```python
from build123d import *

# Parameters (mm, degrees)
F0_W      = 171
F0_H      = 141
F1_DEPTH  = 40
F2_W      = 82.5
F2_H      = 67.5
F3_DEPTH  = 3
F4_W      = 80.5
F4_H      = 65.5
F5_DEPTH  = 3
F6_W      = 82.5
F6_H      = 67.5
F7_DEPTH  = 36
F9_START  = 30
F9_DEPTH  = 6
F11_DEPTH = 39.9
F12_R     = 2.99999
F13_R     = 2.99999
F15_DEPTH = 87.6
F17_DEPTH = 58
F19_DEPTH = 2.5
F20_W     = 34
F20_H     = 30
F20_H_2   = 5
F21_DEPTH = 1.5
F22_W     = 22
F22_H     = 36
F23_DEPTH = 1
F25_DEPTH = 107.7
F27_DEPTH = 2
F29_DEPTH = 18
F31_DEPTH = 6
F33_DEPTH = 6


# Not quite as in the source:
# - a fillet or chamfer is up to 0.001 mm smaller than in the source, because OpenCascade refuses the exact size


with BuildPart() as f1:
    # F0 (on Front) → F1 (new body)
    with BuildSketch(Plane.XZ):
        with Locations((85.5, 70.5)):
            Rectangle(F0_W, F0_H)
    extrude(amount=F1_DEPTH)

    # F2 (on face) → F3 (cut)
    with BuildSketch(Plane.XZ.offset(40)):
        with Locations((126.75, 104.25)):
            Rectangle(F2_W, F2_H)
        with Locations((44.25, 104.25)):
            Rectangle(F2_W, F2_H)
        with Locations((126.75, 36.75)):
            Rectangle(F2_W, F2_H)
        with Locations((44.25, 36.75)):
            Rectangle(F2_W, F2_H)
    extrude(amount=-F3_DEPTH, mode=Mode.SUBTRACT)

    # F4 (on face) → F5 (cut)
    with BuildSketch(Plane.XZ.offset(37)):
        with Locations((45.25, 103.25)):
            Rectangle(F4_W, F4_H)
        with Locations((125.75, 103.25)):
            Rectangle(F4_W, F4_H)
        with Locations((125.75, 37.75)):
            Rectangle(F4_W, F4_H)
        with Locations((45.25, 37.75)):
            Rectangle(F4_W, F4_H)
    extrude(amount=-F5_DEPTH, mode=Mode.SUBTRACT)

    # F6 (on face) → F7 (cut)
    with BuildSketch(Plane.XZ.offset(37)):
        with Locations((126.75, 104.25)):
            Rectangle(F6_W, F6_H)
        with Locations((44.25, 104.25)):
            Rectangle(F6_W, F6_H)
        with Locations((126.75, 36.75)):
            Rectangle(F6_W, F6_H)
        with Locations((44.25, 36.75)):
            Rectangle(F6_W, F6_H)
    extrude(amount=-F7_DEPTH, mode=Mode.SUBTRACT)

    # F8 (on face) → F9 (join)
    with BuildSketch(Plane.XZ.offset(1).offset(F9_START)):
        Polygon((3, 138), (3, 70.5), (6, 70.5), (6, 135), (85.5, 135), (85.5, 138), align=None)
        Polygon((3, 70.5), (3, 3), (85.5, 3), (85.5, 6), (6, 6), (6, 70.5), align=None)
        Polygon((85.5, 6), (85.5, 3), (168, 3), (168, 70.5), (165, 70.5), (165, 6), align=None)
        Polygon((165, 70.5), (168, 70.5), (168, 138), (85.5, 138), (85.5, 135), (165, 135), align=None)
    extrude(amount=F9_DEPTH)

    # F10 (on face) → F11 (cut)
    with BuildSketch(Plane.YZ.offset(171)):
        Polygon((-13, 121), (-13, 106), (-5, 106), (-5, 113.5), (-5, 121), (-9, 121), align=None)
    extrude(amount=-F11_DEPTH, mode=Mode.SUBTRACT)

    # F12 (radius 3 in the source; OpenCascade refuses exactly that, so slightly less here)
    f12_edges = [f1.edges().sort_by_distance(p)[0] for p in [
        (171, -40, 70.5),
    ]]
    fillet(f12_edges, radius=F12_R)

    # F13 (radius 3 in the source; OpenCascade refuses exactly that, so slightly less here)
    f13_edges = [f1.edges().sort_by_distance(p)[0] for p in [
        (0, -40, 70.5),
    ]]
    fillet(f13_edges, radius=F13_R)

    # F14 (on face) → F15 (cut)
    with BuildSketch(Plane.YZ.offset(171)):
        Polygon((-10.5, 78), (-10.5, 69), (-5.5, 69), (-5.5, 73.5), (-5.5, 78), (-8, 78), align=None)
    extrude(amount=-F15_DEPTH, mode=Mode.SUBTRACT)

    # F16 (on face) → F17 (cut)
    with BuildSketch(Plane.YZ.offset(171)):
        Polygon((-17.5, 66.5), (-17.5, 56.5), (-5.5, 56.5), (-5.5, 61.5), (-5.5, 66.5), (-11.5, 66.5), align=None)
    extrude(amount=-F17_DEPTH, mode=Mode.SUBTRACT)

    # F18 (on face) → F19 (join)
    with BuildSketch(Plane.XZ.offset(1)):
        Polygon((134, 138), (131, 138), (131, 3), (134, 3), (134, 70.5), (134, 92), (134, 102), align=None)
        Polygon((151, 102), (134, 102), (134, 92), (168, 92), (168, 102), align=None)
    extrude(amount=F19_DEPTH)

    # F20 (on face) → F21 (join)
    with BuildSketch(Plane.XZ.offset(1)):
        with Locations((151, 77)):
            Rectangle(F20_W, F20_H)
        with Locations((151, 54.5)):
            Rectangle(F20_W, F20_H_2)
    extrude(amount=F21_DEPTH)

    # F22 (on face) → F23 (join)
    with BuildSketch(Plane.XZ.offset(1)):
        with Locations((157, 120)):
            Rectangle(F22_W, F22_H)
    extrude(amount=F23_DEPTH)

    # F24 (on face) → F25 (cut)
    with BuildSketch(Plane.YZ.offset(171)):
        Polygon((-18, 39), (-18, 18), (-11.5, 18), (-5, 18), (-5, 28.5), (-5, 39), align=None)
    extrude(amount=-F25_DEPTH, mode=Mode.SUBTRACT)

    # F26 (on face) → F27 (join)
    with BuildSketch(Plane.XZ.offset(1)):
        Polygon((168, 18), (168, 38), (153, 38), (153, 18), (160.5, 18), align=None)
    extrude(amount=F27_DEPTH)

    # F28 (on face) → F29 (join)
    with BuildSketch(Plane.XZ.offset(1)):
        Polygon((60, 53), (60, 28), (60, 3), (63, 3), (63, 53), align=None)
        Polygon((63, 75), (3, 75), (3, 72), (33, 72), (63, 72), align=None)
    extrude(amount=F29_DEPTH)

    # F30 (on face) → F31 (cut)
    with BuildSketch(Plane.XZ.offset(40)):
        with BuildLine():
            Line((10.05, 139.5), (9, 139.5))
            ThreePointArc((9, 139.5), (10.05, 138.45), (11.1, 139.5))
            Line((11.1, 139.5), (10.05, 139.5))
        make_face()
        with BuildLine():
            ThreePointArc((160.95, 140.55), (160.2075378798, 140.2424621202), (159.9, 139.5))
            Line((159.9, 139.5), (160.95, 139.5))
            Line((160.95, 139.5), (160.95, 140.55))
        make_face()
        with BuildLine():
            Line((160.95, 139.5), (159.9, 139.5))
            ThreePointArc((159.9, 139.5), (160.95, 138.45), (162, 139.5))
            Line((162, 139.5), (160.95, 139.5))
        make_face()
        with BuildLine():
            ThreePointArc((86.55, 139.5), (85.5, 140.55), (84.45, 139.5))
            Line((84.45, 139.5), (86.55, 139.5))
        make_face()
        with BuildLine():
            Line((86.55, 139.5), (84.45, 139.5))
            ThreePointArc((84.45, 139.5), (85.5, 138.45), (86.55, 139.5))
        make_face()
        with BuildLine():
            ThreePointArc((10.05, 140.55), (9.3075378798, 140.2424621202), (9, 139.5))
            Line((9, 139.5), (10.05, 139.5))
            Line((10.05, 139.5), (10.05, 140.55))
        make_face()
        with BuildLine():
            Line((10.05, 139.5), (11.1, 139.5))
            ThreePointArc((11.1, 139.5), (10.7924621202, 140.2424621202), (10.05, 140.55))
            Line((10.05, 140.55), (10.05, 139.5))
        make_face()
        with BuildLine():
            ThreePointArc((162, 139.5), (161.6924621202, 140.2424621202), (160.95, 140.55))
            Line((160.95, 140.55), (160.95, 139.5))
            Line((160.95, 139.5), (162, 139.5))
        make_face()
    extrude(amount=-F31_DEPTH, mode=Mode.SUBTRACT)

    # F32 (on face) → F33 (cut)
    with BuildSketch(Plane.XZ.offset(40)):
        with BuildLine():
            Line((10, 1.5), (9, 1.5))
            ThreePointArc((9, 1.5), (10, 0.5), (11, 1.5))
            Line((11, 1.5), (10, 1.5))
        make_face()
        with BuildLine():
            ThreePointArc((161, 2.5), (160.2928932188, 2.2071067812), (160, 1.5))
            Line((160, 1.5), (161, 1.5))
            Line((161, 1.5), (161, 2.5))
        make_face()
        with BuildLine():
            Line((161, 1.5), (160, 1.5))
            ThreePointArc((160, 1.5), (161, 0.5), (162, 1.5))
            Line((162, 1.5), (161, 1.5))
        make_face()
        with BuildLine():
            ThreePointArc((86.5, 1.5), (85.5, 2.5), (84.5, 1.5))
            Line((84.5, 1.5), (86.5, 1.5))
        make_face()
        with BuildLine():
            Line((86.5, 1.5), (84.5, 1.5))
            ThreePointArc((84.5, 1.5), (85.5, 0.5), (86.5, 1.5))
        make_face()
        with BuildLine():
            ThreePointArc((10, 2.5), (9.2928932188, 2.2071067812), (9, 1.5))
            Line((9, 1.5), (10, 1.5))
            Line((10, 1.5), (10, 2.5))
        make_face()
        with BuildLine():
            Line((10, 1.5), (11, 1.5))
            ThreePointArc((11, 1.5), (10.7071067812, 2.2071067812), (10, 2.5))
            Line((10, 2.5), (10, 1.5))
        make_face()
        with BuildLine():
            ThreePointArc((162, 1.5), (161.7071067812, 2.2071067812), (161, 2.5))
            Line((161, 2.5), (161, 1.5))
            Line((161, 1.5), (162, 1.5))
        make_face()
    extrude(amount=-F33_DEPTH, mode=Mode.SUBTRACT)


solid = f1.part
```
Model file for the job. Use its own axes, mm. A direction names the side the tool comes from. Round coordinates to 2 decimals unless told otherwise and drop trailing zeros. Order: outer loops, then holes, each group sorted by start corner. A loop starts at its lowest first (then second) coordinate and runs counter-clockwise, first axis right, second up. Notation, with made-up numbers: (-30.5, 7.5) -> (-0.5, 7.5) arc R19 ccw to (-0.5, 19.5) -> close; hole circle Ø5 at (32, 8). An arc over 180 degrees is marked (long way). Use one line per item in the form item = value.
Item 1: Tool access for faces 1 (the face through (87, -34, 6)), 2 (the face through (160, -3, 28)), 3 (the face through (84, -20, 0)): list every direction of +Z, -Z, +X, -X, +Y, -Y with a clear straight run to the whole face (end or side of a thin tool).
Returned:
face_1 = -Y
face_2 = none
face_3 = -Z, +X, -X, +Y, -Y
Item 2: Flat gauge pins, fed straight in: pin 1 Ø1 at (y, z) = (-13, 20) entering from +X; pin 2 Ø1 at (x, z) = (85.5, 139.5) entering from -Y; pin 3 Ø1.5 at (x, z) = (169, 73.5) entering from -Y. Where does each tip first touch, or does it go through?
Returned:
pin_1 = 63
pin_2 = -34
pin_3 = -39.99
Item 3: Drill centre lines: line 1 (Z direction, x = 60.5, y = -5); line 2 (Z direction, x = 32, y = -11.5); line 3 (Z direction, x = 85.5, y = -36.6). Where is each one in solid material? Low to high.
Returned:
line_1 = 0 to 53, 72 to 75, 138 to 141
line_2 = 0 to 3, 72 to 75, 138 to 141
line_3 = 0 to 0.5, 2.5 to 6, 135 to 138.45, 140.55 to 141
Item 4: Cut at B-B, the plane x = 20.5. Write the cut outline in (y, z), and give its area (3 significant figures).
Returned:
outline = (-40, 0) -> (0, 0) -> (0, 141) -> (-40, 141) -> (-40, 138) -> (-37, 138) -> (-37, 135) -> (-31, 135) -> (-31, 138) -> (-1, 138) -> (-1, 75) -> (-19, 75) -> (-19, 72) -> (-1, 72) -> (-1, 3) -> (-31, 3) -> (-31, 6) -> (-37, 6) -> (-37, 3) -> (-40, 3) -> close
area = 465 mm^2
Item 5: Pull direction X, two halves, no side cores. Call faces 4 (the face through (84, -20, 141)), 5 (the face through (140, -1, 120)): released by +X, released by -X, zero draft, split by the parting line, or undercut.
Returned:
face_4 = zero draft
face_5 = undercut
